Work out the finished part from the listing and answer in its coordinate system (mm). Give positions to 0.01 mm unless a question says otherwise; leave off trailing zeros. Loops run counter-clockwise (first coordinate to the right, second up) from the corner with the lowest first, then second, coordinate; pieces in that order, holes last. Notation, with made-up numbers: (55.5, 23.25) - (113.5, 23.25) arc R26 cw to (113.5, 61.25) - close; hole circle Ø7 at (54, 75.5). An arc over 180 degrees is marked (long way). One line per item, written item: value.
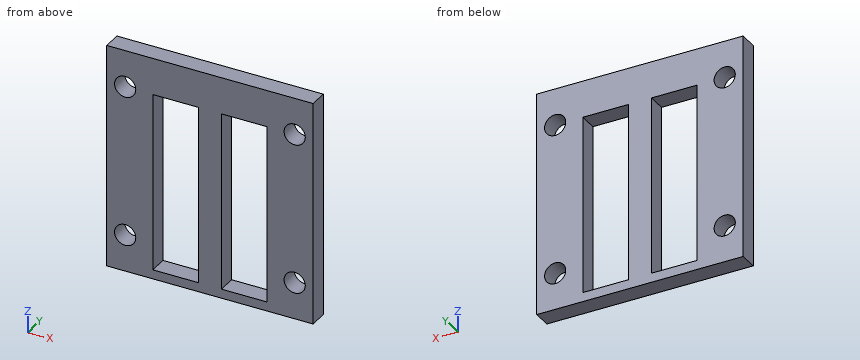
from build123d import *

# Parameters (mm, degrees)
F0_W     = 1.2
F0_H     = 1
F0_W_2   = 1.5
F0_W_3   = 4
F0_H_2   = 2
F0_R     = 1.15
F0_W_4   = 1
F0_H_3   = 4
F0_H_4   = 12.4
F0_W_5   = 4.95
F1_DEPTH = 2


with BuildPart() as f1:
    # F0 (on Front) → F1 (new body)
    with BuildSketch(Plane.XZ):
        with Locations((16.8, 0.5)):
            Rectangle(F0_W, F0_H)
        with Locations((15.45, 0.5)):
            Rectangle(F0_W_2, F0_H)
        Polygon((14.7, 0), (14.7, 1), (12.45, 1), (11.2, 1), (9.95, 1), (7.7, 1), (7.7, 0), align=None)
        Polygon((17.4, 20.4), (17.4, 1), (17.4, 0), (18.4, 0), (18.4, 2), (18.4, 6), (18.4, 18.4), (18.4, 20.4), align=None)
        with Locations((6.95, 0.5)):
            Rectangle(F0_W_2, F0_H)
        with Locations((20.4, 1)):
            Rectangle(F0_W_3, F0_H_2)
        Polygon((18.4, 22.4), (18.4, 20.4), (18.4, 18.4), (22.4, 18.4), (22.4, 22.4), align=None)
        with Locations((20.4, 20.4)):
            Circle(F0_R, mode=Mode.SUBTRACT)
        with Locations((17.9, 23.4)):
            Rectangle(F0_W_4, F0_H_2)
        Polygon((12.45, 22.4), (17.4, 22.4), (17.4, 24.4), (11.2, 24.4), (11.2, 22.4), align=None)
        with Locations((5.6, 0.5)):
            Rectangle(F0_W, F0_H)
        with Locations((20.4, 4)):
            Rectangle(F0_W_3, F0_H_3)
        with Locations((20.4, 4)):
            Circle(F0_R, mode=Mode.SUBTRACT)
        with Locations((20.4, 12.2)):
            Rectangle(F0_W_3, F0_H_4)
        with Locations((20.4, 23.4)):
            Rectangle(F0_W_3, F0_H_2)
        Polygon((4, 0), (5, 0), (5, 1), (5, 20.4), (4, 20.4), (4, 18.4), (4, 6), (4, 2), align=None)
        Polygon((9.95, 22.4), (11.2, 22.4), (11.2, 24.4), (5, 24.4), (5, 22.4), align=None)
        with Locations((2, 1)):
            Rectangle(F0_W_3, F0_H_2)
        with Locations((4.5, 23.4)):
            Rectangle(F0_W_4, F0_H_2)
        with Locations((2, 4)):
            Rectangle(F0_W_3, F0_H_3)
        with Locations((2, 4)):
            Circle(F0_R, mode=Mode.SUBTRACT)
        Polygon((4, 18.4), (4, 20.4), (4, 22.4), (0, 22.4), (0, 18.4), align=None)
        with Locations((2, 20.4)):
            Circle(F0_R, mode=Mode.SUBTRACT)
        with Locations((2, 23.4)):
            Rectangle(F0_W_3, F0_H_2)
        with Locations((2, 12.2)):
            Rectangle(F0_W_3, F0_H_4)
        Polygon((11.2, 1), (12.45, 1), (12.45, 20.4), (11.2, 20.4), (9.95, 20.4), (9.95, 1), align=None)
        with Locations((7.475, 21.4)):
            Rectangle(F0_W_5, F0_H_2)
        with Locations((4.5, 21.4)):
            Rectangle(F0_W_4, F0_H_2)
        Polygon((11.2, 20.4), (12.45, 20.4), (12.45, 22.4), (11.2, 22.4), (9.95, 22.4), (9.95, 20.4), align=None)
        with Locations((17.9, 21.4)):
            Rectangle(F0_W_4, F0_H_2)
        with Locations((14.925, 21.4)):
            Rectangle(F0_W_5, F0_H_2)
    extrude(amount=F1_DEPTH)


solid = f1.part
1. Section A-A (x = 5.5) is taken. Write down the section's boundary in (y, z).
Output:
outline: (-2, 0) - (0, 0) - (0, 1) - (-2, 1) - close; (-2, 20.4) - (0, 20.4) - (0, 24.4) - (-2, 24.4) - close
2. Find the intervals of material crossed by line 1 along Z through (x, y) = (20.4, -0.65); line 2 along X through (y, z) = (-0.6, 14), in increasing order.
Output:
line 1: z = 0 to 2.85, 5.15 to 19.25, 21.55 to 24.4
line 2: x = 0 to 5, 9.95 to 12.45, 17.4 to 22.4
3. Section D-D (x = 20.4) is taken. Write down the section's boundary in (y, z).
Output:
outline: (-2, 0) - (0, 0) - (0, 2.85) - (-2, 2.85) - close; (-2, 5.15) - (0, 5.15) - (0, 19.25) - (-2, 19.25) - close; (-2, 21.55) - (0, 21.55) - (0, 24.4) - (-2, 24.4) - close
4. Section C-C (z = 16) is taken. Write down the section's boundary in (x, y).
Output:
outline: (0, -2) - (5, -2) - (5, 0) - (0, 0) - close; (9.95, -2) - (12.45, -2) - (12.45, 0) - (9.95, 0) - close; (17.4, -2) - (22.4, -2) - (22.4, 0) - (17.4, 0) - close
5. Section B-B (y = -1.6) is taken. Write down the section's boundary in (x, z), and give its area (3 significant figures).
Output:
outline: (0, 0) - (22.4, 0) - (22.4, 24.4) - (0, 24.4) - close; hole circle Ø2.3 at (2, 4); hole circle Ø2.3 at (2, 20.4); hole (5, 1) - (9.95, 1) - (9.95, 20.4) - (5, 20.4) - close; hole (12.45, 1) - (17.4, 1) - (17.4, 20.4) - (12.45, 20.4) - close; hole circle Ø2.3 at (20.4, 4); hole circle Ø2.3 at (20.4, 20.4)
area: 338 mm²
6. A flat-ended cylindrical pin translates along its axis: pin 1 Ø1.4 at (x, z) = (2, 4) entering from -Y. Find the tip coordinate at first contact, or state that the pin passes through.
Output:
pin 1: passes through
